```python
from build123d import *

# Parameters (mm, degrees)
SKETCH1_R               = 6.35
SKETCH1_R_2             = 5.461
EXTRUDE1_DEPTH          = 85.725
SKETCH2_R               = 2
CUT_EXTRUDE1_DEPTH      = 38.1
CUT_EXTRUDE1_DEPTH_BACK = 38.1


with BuildPart() as part:
    # Sketch1 → Extrude1 (new body)
    with BuildSketch(Plane.XY):
        Circle(SKETCH1_R)
        Circle(SKETCH1_R_2, mode=Mode.SUBTRACT)
    extrude(amount=EXTRUDE1_DEPTH)

    # Sketch2 → Cut-Extrude1 (cut, two sides)
    with BuildSketch(Plane(origin=(0, 0, 0), x_dir=(1, 0, 0), z_dir=(0, 1, 0))) as cut_extrude1_sk:
        with Locations(Location((0, -9.525, 0), (0, 0, 270))):  # turned: the seam where the file's is
            Circle(SKETCH2_R)
        with Locations(Location((0, -76.2, 0), (0, 0, 270))):  # turned: the seam where the file's is
            Circle(SKETCH2_R)
    extrude(amount=CUT_EXTRUDE1_DEPTH, mode=Mode.SUBTRACT)
    extrude(cut_extrude1_sk.sketch, amount=-CUT_EXTRUDE1_DEPTH_BACK, mode=Mode.SUBTRACT)


solid = part.part
```
Work out the finished part from the listing and answer in its coordinate system (mm). Give positions to 0.01 mm unless a question says otherwise; leave off trailing zeros. Order: outer loops, then holes, each group sorted by start corner. A loop starts at its lowest first (then second) coordinate and runs counter-clockwise, first axis right, second up. Notation, with made-up numbers: M 44.5,-4.5 L 86.5,-4.5 A19 cw 86.5,24.5 Z; hole C 31,-15 d5. An arc over 180 degrees is marked long. Return JSON: item names as keys, results as strings.
1) Section B-B, the plane x = 0 is taken. Write down the section's boundary in (y, z) (3 decimals), plus the area to 3 significant figures.
Resolved:
{"outline": "M -6.35,0 L -5.461,0 L -5.461,7.525 L -6.35,7.525 Z; M -6.35,11.525 L -5.461,11.525 L -5.461,74.2 L -6.35,74.2 Z; M -6.35,78.2 L -5.461,78.2 L -5.461,85.725 L -6.35,85.725 Z; M 5.461,0 L 6.35,0 L 6.35,7.525 L 5.461,7.525 Z; M 5.461,11.525 L 6.35,11.525 L 6.35,74.2 L 5.461,74.2 Z; M 5.461,78.2 L 6.35,78.2 L 6.35,85.725 L 5.461,85.725 Z", "area": "138 mm^2"}
2) Section A-A, the plane y = 0 is taken. Write down the section's boundary in (x, z) (3 decimals), plus the area to 3 significant figures.
Resolved:
{"outline": "M -6.35,0 L -5.461,0 L -5.461,85.725 L -6.35,85.725 Z; M 5.461,0 L 6.35,0 L 6.35,85.725 L 5.461,85.725 Z", "area": "152 mm^2"}
3) Section C-C, the plane z = 76.2 is taken. Write down the section's boundary in (x, y), plus the area to 3 significant figures.
Resolved:
{"outline": "M -2,-6.03 L -2,-5.08 A5.46 cw -2,5.08 L -2,6.03 A6.35 ccw Z; M 2,-6.03 A6.35 ccw 2,6.03 L 2,5.08 A5.46 cw 2,-5.08 Z", "area": "25.7 mm^2"}
4) Straight lines are drawn through the part: line 1 along Z through (x, y) = (0, 5.75) (3 decimals); line 2 along Y through (x, z) = (0, 35.5); line 3 along Y through (x, z) = (-1, 73). For each, find the intervals that lie inside material, in ascending order. Write a range as [from, to].
Resolved:
{"line 1": "[0, 7.525], [11.525, 74.2], [78.2, 85.725]", "line 2": "[-6.35, -5.46], [5.46, 6.35]", "line 3": "[-6.27, -5.37], [5.37, 6.27]"}
5) For a pull along X with two mould halves and no side action, classify faces 1 (the cylindrical face through (5.21, 1.64, 42.26)), 2 (the cylindrical face through (-1.38, -6.2, 42.26)), 3 (the flat face through (3, 5, 85.725)) as +X half, -X half, draft (parallel to the pull), parting line (faces both ways), or undercut.
Resolved:
{"face 1": "undercut", "face 2": "parting line", "face 3": "draft"}
6) Section D-D, the plane z = 17 is taken. Write down the section's boundary in (x, y), plus the area to 3 significant figures.
Resolved:
{"outline": "C 0,0 d12.7; hole C 0,0 d10.92", "area": "33.0 mm^2"}
7) Each of these flat-tipped pins is pushed along its axis until it touches: pin 1 (4.5 mm diameter, centred on x = 0, z = 9.525, fed in from +Y); pin 2 (3 mm diameter, centred on x = -4, z = 39.5, fed in from +Y); pin 3 (4 mm diameter, centred on x = -4, z = 12.5, fed in from +Y); pin 4 (2 mm diameter, centred on y = 2, z = 29.5, fed in from -X). Where does it stop, or does it pass through?
Resolved:
{"pin 1": "y = 6.35", "pin 2": "y = 5.84", "pin 3": "y = 6.03", "pin 4": "x = -6.27"}
